```python
from build123d import *

# Parameters (mm, degrees)
F2_R     = 4.7625
F3_DEPTH = 19.05


with BuildPart() as f3:
    # F2 (on Right) → F3 (new body)
    with BuildSketch(Plane.YZ):
        Polygon((-1407.371283, 324.033141), (-1422.397137, 303.945631), (-1415.061831, 223.747462), (-1388.655186, 197.829768), (-1286.451459, 181.692332), (-1293.786645, 206.142992), (-1294.275641, 267.025113), (-1270.06948, 287.563682), (-1269.580483, 311.280817), (-1316.281199, 327.418238), align=None)
        with Locations((-1392.702985, 315.051372)):
            Circle(F2_R, mode=Mode.SUBTRACT)
        with Locations((-1297.021795, 298.678095)):
            Circle(F2_R, mode=Mode.SUBTRACT)
    extrude(amount=F3_DEPTH)


solid = f3.part
```
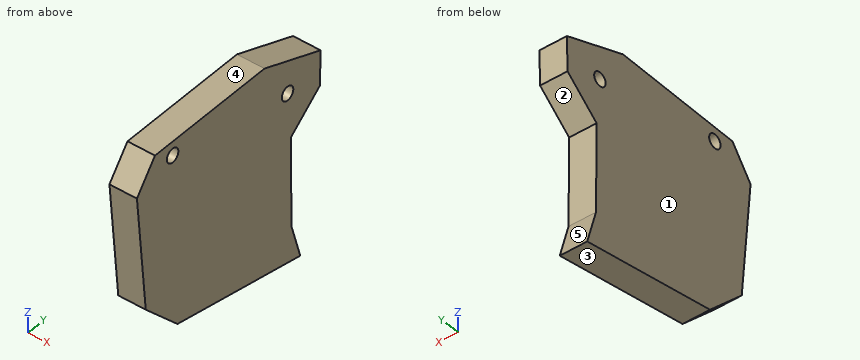
Could you check a few things on this model? Use its own coordinates, in mm. Face numbers are marked on the shaded views. A direction names the side the tool comes from. Round coordinates to 2 decimals unless told otherwise and drop trailing zeros. Loops run counter-clockwise (first coordinate to the right, second up) from the corner with the lowest first, then second, coordinate; pieces in that order, holes last. Notation, with made-up numbers: (22.5, 21.25) - (72.5, 21.25) arc R20 ccw to (72.5, 31.25) - close; hole circle Ø11 at (35, -11.75). An arc over 180 degrees is marked (long way). Answer in a Markdown table with one row per item. Add a question column.
(1) If we section it at C-C (y = -1336): Please give me the cut outline in (x, z).
(2) For the marked faces 1 and 2, which set-ups out of +Z, -Z, +X, -X, +Y, -Y let a thin tool reach every point of the face, with its end or its side?
(3) If we section it at A-A (x = 6.25): Please give me the cut outline in (y, z) (1 decimal), plus the area to 3 significant figures.
(4) If we section it at D-D (z = 201): Please give me the cut outline in (x, y).
(5) If we section it at B-B (z = 317.5): Please give me the cut outline in (x, y).
(6) If we mould it in two halves opening along Z, with no side actions, what happens to the marked faces 3, 4 and 5? For each: pulls with the +Z half, pulls with the -Z half, needs draft (parallel to the pull), parting line crosses it, or undercut.
(7) I'm going to push flat-ended pins straight in: pin 1 (5 mm diameter, centred on x = 3, z = 303.5, fed in from +Y); pin 2 (2 mm diameter, centred on x = 6, z = 266, fed in from +Y); pin 3 (6 mm diameter, centred on x = 9, y = -1292.5, fed in from +Z). Where does each tip first touch, or does it pass through?
(8) I need wall thicknesses on line 1 along Z through (x, y) = (7, -1391.5); line 2 along Z through (x, y) = (4.25, -1397); line 3 along Z through (x, y) = (12.5, -1322.5). Which ranges of each line are inside material? Lowest first, please.
Model answer:
| question | item | result |
|---|---|---|
| 1 | outline | (0, 189.52) - (19.05, 189.52) - (19.05, 326.69) - (0, 326.69) - close |
| 2 | face 1 | +Z, -Z, -X, +Y, -Y |
| 2 | face 2 | +X, -X, +Y |
| 3 | outline | (-1422.4, 303.9) - (-1415.1, 223.7) - (-1388.7, 197.8) - (-1286.5, 181.7) - (-1293.8, 206.1) - (-1294.3, 267) - (-1270.1, 287.6) - (-1269.6, 311.3) - (-1316.3, 327.4) - (-1407.4, 324) - close; hole circle Ø9.5 at (-1392.7, 315.1); hole circle Ø9.5 at (-1297, 298.7) |
| 3 | area | 16,900 mm² |
| 4 | outline | (0, -1391.89) - (19.05, -1391.89) - (19.05, -1292.24) - (0, -1292.24) - close |
| 5 | outline | (0, -1412.26) - (19.05, -1412.26) - (19.05, -1396.79) - (0, -1396.79) - close; (0, -1388.62) - (19.05, -1388.62) - (19.05, -1287.58) - (0, -1287.58) - close |
| 6 | face 3 | pulls with the -Z half |
| 6 | face 4 | pulls with the +Z half |
| 6 | face 5 | undercut |
| 7 | pin 1 | stops at y = -1269.69 |
| 7 | pin 2 | stops at y = -1294.26 |
| 7 | pin 3 | stops at z = 320.24 |
| 8 | line 1 | z = 200.62 to 310.44, 319.66 to 324.62 |
| 8 | line 2 | z = 206.02 to 313, 317.1 to 324.42 |
| 8 | line 3 | z = 187.38 to 327.19 |
